from build123d import *

# Parameters (mm, degrees)
EXTRUDE_3_DEPTH     = 10
SKETCH_4_W          = 2.5
SKETCH_4_H          = 21.5
EXTRUDE_4_DEPTH     = 1.5
SKETCH_5_R          = 0.85
EXTRUDE_5_DEPTH     = 6.9
CUT_EXTRUDE_START   = 2
SKETCH_6_W          = 3.85
SKETCH_6_H          = 12.8
CUT_EXTRUDE_1_DEPTH = 25.397158938


with BuildPart() as part:
    # Эскиз3 → Бобышка-Вытянуть3 (new body)
    with BuildSketch(Plane(origin=(0, 0, 0), x_dir=(0, 0, -1), z_dir=(1, 0, 0))):
        Polygon((0, 0), (-21.5, 0), (-21.5, 11.6), (-20, 11.6), (-20, 1.5), (0, 1.5), align=None)
    extrude(amount=-EXTRUDE_3_DEPTH)

    # Эскиз4 → Бобышка-Вытянуть4 (add)
    with BuildSketch(Plane(origin=(0, 0, 0), x_dir=(1, 0, 0), z_dir=(0, 1, 0))):
        with Locations((-8.75, -10.75)):
            Rectangle(SKETCH_4_W, SKETCH_4_H)
    extrude(amount=-EXTRUDE_4_DEPTH)

    # Эскиз5 → Бобышка-Вытянуть5 (add)
    with BuildSketch(Plane(origin=(0, 0, 0), x_dir=(1, 0, 0), z_dir=(0, 1, 0))):
        with Locations(Location((-5.8, -7.15, 0), (0, 0, 270))):
            Circle(SKETCH_5_R)
        with Locations(Location((-5.8, -13.65, 0), (0, 0, 270))):
            Circle(SKETCH_5_R)
        Polygon((-7.5, 0), (-3.65, 0), (0, 0), (0, -4), (-3.65, -4), (-7.5, -4), (-7.5, -4.75), (-10, -4.75), (-10, 0), align=None)
        Polygon((-7.5, -21.5), (-3.65, -21.5), (-3.65, -16.8), (-7.5, -16.8), (-7.5, -16.05), (-10, -16.05), (-10, -21.5), align=None)
    extrude(amount=-EXTRUDE_5_DEPTH)

    # Эскиз6 → Вырез-Вытянуть1 (cut, through all)
    with BuildSketch(Plane.XZ.offset(CUT_EXTRUDE_START)):
        with Locations((-5.575, 10.4)):
            Rectangle(SKETCH_6_W, SKETCH_6_H)
    extrude(amount=CUT_EXTRUDE_1_DEPTH, mode=Mode.SUBTRACT)


solid = part.part
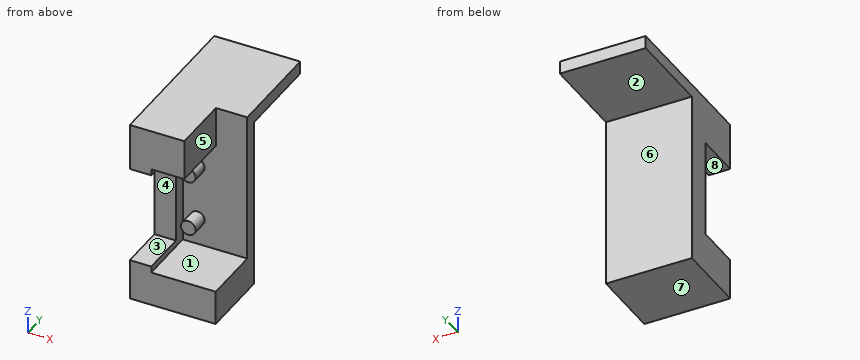
Read the model definition and answer for the solid it produces. Units are mm, in the model's axes. Face numbers are marked on the shaded views. A direction names the side the tool comes from. Round coordinates to 2 decimals unless told otherwise and drop trailing zeros. Write each loop counter-clockwise with the first axis right and the second up, starting at its lowest first coordinate (ties: lowest second). Pieces come first, ordered by that corner, then holes. Notation, with made-up numbers: M 67,-4 L 91,-4 A28 ccw 91,35 Z; hole C 49.5,41.25 d7. An arc over 180 degrees is marked long. Use a Markdown table: item, result.
1) For a pull along Z with two mould halves and no side action, classify the marked faces 6, 7 and 8 as pulls with the +Z half, pulls with the -Z half, needs draft (parallel to the pull), parting line crosses it, or undercut.
Answers follow:
| item | result |
|---|---|
| face 6 | needs draft |
| face 7 | pulls with the -Z half |
| face 8 | undercut |
2) The part is cut by section C-C (x = -7.25). Write down the section's boundary in (y, z), plus the area to 3 significant figures.
Answers follow:
| item | result |
|---|---|
| outline | M -6.9,0 L 1.5,0 L 1.5,20 L 11.6,20 L 11.6,21.5 L -6.9,21.5 L -6.9,16.8 L 0,16.8 L 0,4 L -6.9,4 Z |
| area | 107 mm2 |
3) The part is cut by section D-D (y = -0.25). Write down the section's boundary in (x, z).
Answers follow:
| item | result |
|---|---|
| outline | M -10,0 L 0,0 L 0,4 L -7.5,4 L -7.5,16.8 L -3.65,16.8 L -3.65,21.5 L -10,21.5 Z; C -5.8,7.15 d1.7; C -5.8,13.65 d1.7 |
4) Straight lines are drawn through the part: line 1 along Z through (x, y) = (-4.25, -3.5); line 2 along Y through (x, z) = (-3.75, 15); line 3 along Z through (x, y) = (-8.5, 10). For each, find the intervals that lie inside material, in ascending order. Write a range as [from, to].
Answers follow:
| item | result |
|---|---|
| line 1 | z = [0, 4], [16.8, 21.5] |
| line 2 | y = [0, 1.5] |
| line 3 | z = [20, 21.5] |
5) Flat-ended cylindrical pins translate along their axes: pin 1 (2 mm diameter, centred on x = -2, z = 10.5, fed in from -Y); pin 2 (1.4 mm diameter, centred on x = -6, z = 7, fed in from -Y); pin 3 (4 mm diameter, centred on y = -4.5, z = 20, fed in from +X). Find the tip coordinate at first contact, or state that the pin passes through.
Answers follow:
| item | result |
|---|---|
| pin 1 | stops at y = 0 |
| pin 2 | stops at y = -2 |
| pin 3 | stops at x = -3.65 |
6) A tool of negligible diameter and unlimited length cuts with its end or side. For the marked faces 1, 2, 3, 4 and 5, from which of +Z, -Z, +X, -X, +Y, -Y can it reach the whole face along a straight path? Write none if from no direction.
Answers follow:
| item | result |
|---|---|
| face 1 | +X, -Y |
| face 2 | -Z, +X, -X, +Y |
| face 3 | +X, -X, -Y |
| face 4 | -X, -Y |
| face 5 | +Z, +X, -Y |
7) The part is cut by section B-B (z = 7.15). Write down the section's boundary in (x, y).
Answers follow:
| item | result |
|---|---|
| outline | M -10,-1.5 L -7.5,-1.5 L -7.5,0 L -6.65,0 L -6.65,-2 L -4.95,-2 L -4.95,0 L 0,0 L 0,1.5 L -10,1.5 Z |
8) The part is cut by section A-A (y = -3). Write down the section's boundary in (x, z), plus the area to 3 significant figures.
Answers follow:
| item | result |
|---|---|
| outline | M -10,0 L 0,0 L 0,4 L -7.5,4 L -7.5,4.75 L -10,4.75 Z; M -10,16.05 L -7.5,16.05 L -7.5,16.8 L -3.65,16.8 L -3.65,21.5 L -10,21.5 Z |
| area | 73.6 mm2 |
